```python
from build123d import *

# Parameters (mm, degrees)
SKETCH1_R                = 6.35
BOSS_EXTRUDE1_DEPTH      = 76.2
BOSS_EXTRUDE2_DEPTH      = 6.35
BOSS_EXTRUDE2_DEPTH_BACK = 6.35
SKETCH2_W                = 13.071299085
SKETCH2_H                = 12.7
CUT_EXTRUDE1_DEPTH       = 6.35
CUT_EXTRUDE1_DEPTH_BACK  = 6.35
SKETCH3_R                = 3.1115


with BuildPart() as part:
    # Sketch1 → Boss-Extrude1 (new body)
    with BuildSketch(Plane.XY):
        with Locations(Location((0, 0, 0), (0, 0, 180))):
            Circle(SKETCH1_R)
    extrude(amount=BOSS_EXTRUDE1_DEPTH)

    # Sketch2 → Boss-Extrude2 (add, two sides: drawn at the far end of the back side and taken through both)
    with BuildSketch(Plane(origin=(0, 0, 0), x_dir=(0, 0, -1), z_dir=(1, 0, 0)).offset(-BOSS_EXTRUDE2_DEPTH_BACK)):
        with Locations((-38.10000004, 0)):
            Rectangle(SKETCH2_W, SKETCH2_H)
    extrude(amount=BOSS_EXTRUDE2_DEPTH + BOSS_EXTRUDE2_DEPTH_BACK)

    # Sketch3 → Cut-Extrude1 (cut, two sides: drawn at the far end of the back side and taken through both)
    with BuildSketch(Plane(origin=(0, 0, 0), x_dir=(0, 0, -1), z_dir=(1, 0, 0)).offset(-CUT_EXTRUDE1_DEPTH_BACK)):
        with Locations((-38.1, 0)):
            Circle(SKETCH3_R)
    extrude(amount=CUT_EXTRUDE1_DEPTH + CUT_EXTRUDE1_DEPTH_BACK, mode=Mode.SUBTRACT)


solid = part.part
```
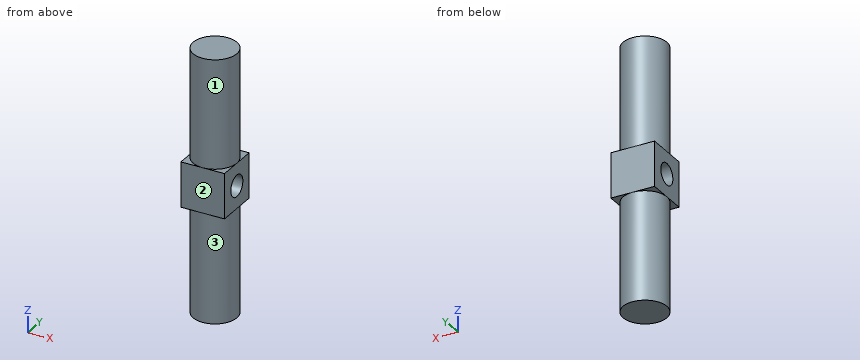
For this review, take the finished solid that the model builds, in its own axes (mm). Face numbers are marked on the shaded views. A direction names the side the tool comes from. Give positions to 0.01 mm unless a question says otherwise; leave off trailing zeros. Write each loop counter-clockwise with the first axis right and the second up, starting at its lowest first coordinate (ties: lowest second). Pieces come first, ordered by that corner, then holes. Notation, with made-up numbers: M 52,-17 L 105,-17 A34 ccw 105,13 Z; hole C -8,13 d10. An arc over 180 degrees is marked long. One line per item, written item: value.
1) For P1, Ø3, axis at y = -3.5, z = 18.5, coming from the -X side; P2, Ø5, axis at x = 3.5, y = -4, coming from the -Z side; P3, Ø5, axis at x = -4, z = 55.5, coming from the +Y side; P4, Ø1.5, axis at y = 2, z = 64, coming from the -X side, all flat-tipped, find the tip position at first contact; note any pin that passes through.
Results are:
P1: stops at x = -6.03
P2: stops at z = 0
P3: stops at y = 6.17
P4: stops at x = -6.23
2) For the marked faces 1, 2 and 3, list the 3-axis set-ups (+Z, -Z, +X, -X, +Y, -Y) from which the entire face can be reached by the end or side of a thin tool; tool diameter is ignored.
Results are:
face 1: +Z
face 2: +Z, -Z, +X, -X, -Y
face 3: -Z
3) For line 1 (Y direction, x = 2, z = 38.1); line 2 (Z direction, x = 5.75, y = -4); line 3 (Z direction, x = 2.5, y = 2.75), list the stretches that pass through material, from the lowest coordinate up. Write a range as from..to.
Results are:
line 1: y = -6.35..-3.11, 3.11..6.35
line 2: z = 31.56..44.64
line 3: z = 0..36.64, 39.56..76.2
4) Take a section at C-C, the plane y = 1. Write out the cut boundary in (x, z), then the cut area to 3 significant figures.
Results are:
outline: M -6.35,31.56 L -6.27,31.56 L -6.27,0 L 6.27,0 L 6.27,31.56 L 6.35,31.56 L 6.35,35.15 L -6.35,35.15 Z; M -6.35,41.05 L 6.35,41.05 L 6.35,44.64 L 6.27,44.64 L 6.27,76.2 L -6.27,76.2 L -6.27,44.64 L -6.35,44.64 Z
area: 883 mm²
5) Take a section at A-A, the plane z = 38.1. Write out the cut boundary in (x, y), then the cut area to 3 significant figures.
Results are:
outline: M -6.35,-6.35 L 6.35,-6.35 L 6.35,-3.11 L -6.35,-3.11 Z; M -6.35,3.11 L 6.35,3.11 L 6.35,6.35 L -6.35,6.35 Z
area: 82.3 mm²
6) Take a section at D-D, the plane z = 30. Write out the cut boundary in (x, y), then the cut area to 3 significant figures.
Results are:
outline: C 0,0 d12.7
area: 127 mm²
7) Take a section at B-B, the plane x = 5. Write out the cut boundary in (y, z), then the cut area to 3 significant figures.
Results are:
outline: M -6.35,31.56 L -3.91,31.56 L -3.91,0 L 3.91,0 L 3.91,31.56 L 6.35,31.56 L 6.35,44.64 L 3.91,44.64 L 3.91,76.2 L -3.91,76.2 L -3.91,44.64 L -6.35,44.64 Z; hole C 0,38.1 d6.22
area: 630 mm²
